Autodesk Inventor part; units mm, degrees
ref_plane "YZ Plane" through (0, 0, 0) normal (1, 0, 0) x (0, 1, 0)
ref_plane "XZ Plane" through (0, 0, 0) normal (0, 1, 0) x (-1, 0, 0)
ref_plane "XY Plane" through (0, 0, 0) normal (0, 0, 1) x (1, 0, 0)
sketch "Sketch1" plane through (0, 0, 0) normal (0, 1, 0) x (-1, 0, 0)
  line L0 (0, 0) -> (38.1, 0)
  line L1 (38.1, -19.05) -> (38.1, -76.2)
  line L2 (38.1, -76.2) -> (0, -76.2)
  line L3 (0, -76.2) -> (0, -19.05)
  arc A0 (38.1, -19.05) -> (0, -19.05) centre (19.05, -19.05) ccw
  dimension "d0" = 38.1
  dimension "d1" = 76.2
extrude "Extrusion1" add sketch "Sketch1" along normal blind 25.4
sketch "Sketch2" plane through (0, 25.4, 0) normal (0, 1, 0) x (1, 0, 0)
  arc A0 (-38.1, 19.05) -> (0, 19.05) centre (-19.05, 19.05) ccw
  circle A1 centre (-19.05, 19.05) radius 19.05
  point P0 (0, 0)
extrude "Extrusion2" add sketch "Sketch2" along normal blind 76.2
sketch "Sketch3" plane through (0, 25.4, 0) normal (0, 1, 0) x (1, 0, 0)
  line L0 (0, 76.2) -> (-38.1, 76.2)
  line L1 (0, 76.2) -> (-38.1, 76.2)
  line L2 (-38.1, 76.2) -> (-38.1, 57.8757)
  line L3 (0, 57.8757) -> (0, 76.2)
  arc A0 (-38.1, 57.8757) -> (0, 57.8757) centre (-19.05, 57.8757) ccw
  point P0 (0, 0)
extrude "Extrusion3" add sketch "Sketch3" along normal blind 139.7
sketch "Sketch4" plane through (0, 165.1, 0) normal (0, 1, 0) x (1, 0, 0)
  circle A0 centre (-19.05, 57.8757) radius 6.35
  arc A1 (-38.1, 57.8757) -> (0, 57.8757) centre (-19.05, 57.8757) ccw
  point P0 (0, 0)
  dimension "d9" = 12.7
extrude "Extrusion4" cut sketch "Sketch4" against normal blind 121.92
properties part number "Actuator new" material "Aluminum 6061"
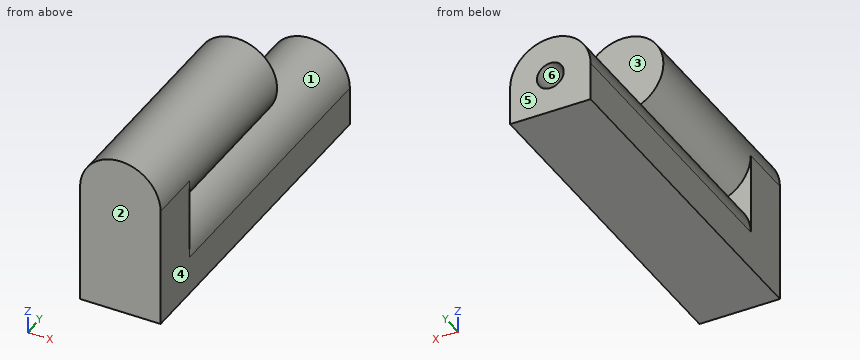
Input: part model. Units: mm. Frame: model coordinates. Face numbers are marked on the shaded views. A direction names the side the tool comes from. Coordinates: 2 decimals unless noted, no trailing zeros. Write each loop counter-clockwise with the first axis right and the second up, starting at its lowest first coordinate (ties: lowest second). Pieces come first, ordered by that corner, then holes.
1) Section B-B on x = -19.05. Output: boundary loops of the cut face in (y, z), and give its area (3 significant figures).
2) Pin query (flat end, axial travel): pin 1 Ø14.5 at (x, z) = (-19.05, -57.88) entering from -Y; pin 2 Ø2 at (x, y) = (-14.5, 70) entering from +Z; pin 3 Ø2 at (y, z) = (67, -36.5) entering from +X; pin 4 Ø4 at (x, z) = (-19.5, -59.5) entering from +Y. Return the tip coordinate at first contact, or that it passes through.
3) Section A-A on y = 46.5. Output: boundary loops of the cut face in (x, z), and give its area (3 significant figures).
4) Mould query, pull axis X, two halves, no side actions, for the marked faces 4, 5 and 6. Classes: pulls with the +X half, pulls with the -X half, needs draft (parallel to the pull), parting line crosses it, or undercut.
5) Section D-D on y = 119. Output: boundary loops of the cut face in (x, z), and give its area (3 significant figures).
6) Set-up query: the marked faces 1, 2 and 3. Return all of +Z, -Z, +X, -X, +Y, -Y with unobstructed straight access to the full face (end or side cutting, diameter ignored); none if empty.
7) Material intervals for line 1 along Z through (x, y) = (-19, 68); line 2 along Z through (x, y) = (-19.05, 133.5); line 3 along Y through (x, z) = (-11, -20), sorted ascending.
8) Section C-C on z = -40.5. Output: boundary loops of the cut face in (x, y), and give its area (3 significant figures).
Check result:
1. outline: (0, -76.2) - (165.1, -76.2) - (165.1, -64.23) - (43.18, -64.23) - (43.18, -51.53) - (165.1, -51.53) - (165.1, -38.83) - (25.4, -38.83) - (25.4, -38.1) - (101.6, -38.1) - (101.6, 0) - (0, 0) - close
1. area: 8,510 mm2
2. pin 1: stops at y = 0
2. pin 2: stops at z = -0.33
2. pin 3: stops at x = -9.44
2. pin 4: stops at y = 43.18
3. outline: (-38.1, -76.2) - (0, -76.2) - (0, -57.88) arc R19.05 ccw to (-38.1, -57.88) - close; circle Ø38.1 at (-19.05, -19.05); hole circle Ø12.7 at (-19.05, -57.88)
3. area: 2,280 mm2
4. face 4: pulls with the +X half
4. face 5: needs draft
4. face 6: undercut
5. outline: (-38.1, -76.2) - (0, -76.2) - (0, -57.88) arc R19.05 ccw to (-38.1, -57.88) - close; hole circle Ø12.7 at (-19.05, -57.88)
5. area: 1,140 mm2
6. face 1: +Y
6. face 2: +Z, -Z, +X, -X, -Y
6. face 3: +Z, +X, -X, +Y
7. line 1: z = -76.2 to -64.23, -51.53 to -38.83, -38.1 to 0
7. line 2: z = -76.2 to -64.23, -51.53 to -38.83
7. line 3: y = 0 to 101.6
8. outline: (-38.1, 0) - (0, 0) - (0, 25.4) - (-11.24, 25.4) - (-11.24, 165.1) - (-26.86, 165.1) - (-26.86, 25.4) - (-38.1, 25.4) - close
8. area: 3,150 mm2
